Check sheet for the modelled part. Datum: model origin and axes. Units: mm. A direction names the side the tool comes from. Give positions to 0.01 mm unless a question says otherwise; leave off trailing zeros. Write each loop counter-clockwise with the first axis right and the second up, starting at its lowest first coordinate (ties: lowest second). Pieces come first, ordered by that corner, then holes.
Autodesk Inventor part; units mm, degrees
ref_plane "XZ Plane" through (0, 0, 0) normal (0, 1, 0) x (-1, 0, 0)
sketch "Sketch1" plane through (0, 0, 0) normal (1, 0, 0) x (0, 1, 0)
  line L0 (-136.2516, 26.0681) -> (-94.6911, -0.9217)
  line L1 (-94.6911, -0.9217) -> (-36.9927, -10.7705)
  line L2 (-36.9927, -10.7705) -> (-22.35, 3.08)
  line L3 (-22.35, 3.08) -> (21.5, 3.08)
  line L4 (21.5, 3.08) -> (21.5, -69)
  line L5 (21.5, -69) -> (-136.2516, -80.5428)
  line L6 (-136.2516, -80.5428) -> (-136.2516, 26.0681)
  line L7 (-20.328, 3.08) -> (15.75, 3.08)
  line L8 (21.5, 2) -> (21.5, -10)
  line L9 (-36.9927, -10.7705) -> (-23.8189, 1.6905)
  line L10 (-136.2516, -70.0311) -> (-136.2516, 7.0311)
  line L11 (-120.3625, 15.7495) -> (-94.6911, -0.9217)
  point P0 (0, 0)
  point P1 (-136.2516, 7.0311)
  dimension "d0" = 46.592
  dimension "d1" = 94.185
  dimension "d2" = 99.687
  dimension "d3" = 57
  dimension "d4" = 157.7516
  dimension "d5" = 21.5
  dimension "d6" = 3.08
  dimension "d7" = 17.5961
  dimension "d8" = 70.385
  dimension "d9" = 16.8414
  dimension "d10" = 52.3454
  dimension "d11" = 1.08
  dimension "d12" = 13.08
  dimension "d13" = 5.75
  dimension "d14" = 41.828
  dimension "d15" = 45.3189
  dimension "d16" = 141.8624
  dimension "d17" = 3.9511
  dimension "d18" = 73.1111
extrude "Extrusion1" add sketch "Sketch1" along normal mid plane 48.9966
properties part number "BaseBoundingBox"
1) Access from +Z, -Z, +X, -X, +Y, -Y to the whole of each face (thin tool, end or side, straight path). Record for faces 5 (the flat face through (-0.34, -56.27, -74.69)), 6 (the flat face through (-0.343, -66.246, -5.777)), 7 (the flat face through (0, -1, 3.08)).
2) Draft check along Y on faces 1 (the flat face through (0, 21.5, -32)), 2 (the flat face through (24.498, -58, -38)), 3 (the flat face through (-0.34, -29.77, -3.94)), 4 (the flat face through (0, -136.252, -28)). Enter one of: +Y half, -Y half, draft (parallel to the pull), parting line (faces both ways), or undercut.
3) Sectioned sample at D-D on y = -3.5. Record the boundary of the cut face in (x, z), then the cut area to 3 significant figures.
4) Sectioned sample at A-A on z = -5. Record the boundary of the cut face in (x, y), then the cut area to 3 significant figures.
5) Sectioned sample at C-C on y = -45.5. Record the boundary of the cut face in (x, z).
6) Scan lines: L1, parallel to Z at x = 22, y = 13; L2, parallel to Z at x = -8, y = -58; L3, parallel to Y at x = -7, z = 5. Record each from-to range of solid material in increasing order.
7) Gauge pin test, flat ends, axial feed: pin 1 (4 mm diameter, centred on x = 19.5, y = -21.5, fed in from -Z); pin 2 (12 mm diameter, centred on x = 1.5, y = -120, fed in from -Z); pin 3 (1.5 mm diameter, centred on x = -1, y = -23, fed in from +Z). Record the tip position at first contact, or that the pin passes through.
8) Sectioned sample at B-B on x = -8. Record the boundary of the cut face in (y, z), then the cut area to 3 significant figures.
Answers below:
1. face 5: -Z, +X, -X, +Y
1. face 6: +Z, +X, -X
1. face 7: +Z, +X, -X, +Y
2. face 1: +Y half
2. face 2: draft
2. face 3: undercut
2. face 4: -Y half
3. outline: (-24.5, -70.83) - (24.5, -70.83) - (24.5, 3.08) - (-24.5, 3.08) - close
3. area: 3,620 mm2
4. outline: (-24.5, -136.25) - (24.5, -136.25) - (24.5, -70.8) - (-24.5, -70.8) - close; (-24.5, -30.89) - (24.5, -30.89) - (24.5, 21.5) - (-24.5, 21.5) - close
4. area: 5,770 mm2
5. outline: (-24.5, -73.9) - (24.5, -73.9) - (24.5, -9.32) - (-24.5, -9.32) - close
6. L1: z = -69.62 to 3.08
6. L2: z = -74.82 to -7.18
6. L3: y = -136.25 to -103.81
7. pin 1: stops at z = -72.29
7. pin 2: stops at z = -79.79
7. pin 3: stops at z = 3.08
8. outline: (-136.25, -80.54) - (21.5, -69) - (21.5, 3.08) - (-22.35, 3.08) - (-36.99, -10.77) - (-94.69, -0.92) - (-136.25, 26.07) - close
8. area: 12,100 mm2
